Could you check a few things on this model? Use its own coordinates, in mm. Face numbers are marked on the shaded views. A direction names the side the tool comes from. Coordinates: 2 decimals unless noted, no trailing zeros. Order: outer loops, then holes, each group sorted by start corner. A loop starts at its lowest first (then second) coordinate and runs counter-clockwise, first axis right, second up. Notation, with made-up numbers: M 28,-27.75 L 35,-27.75 A8 ccw 35,-15.75 Z; hole C -35.75,-27 d9. An arc over 180 degrees is marked long. One line per question, with ' | ' between items. Start each with the question number.
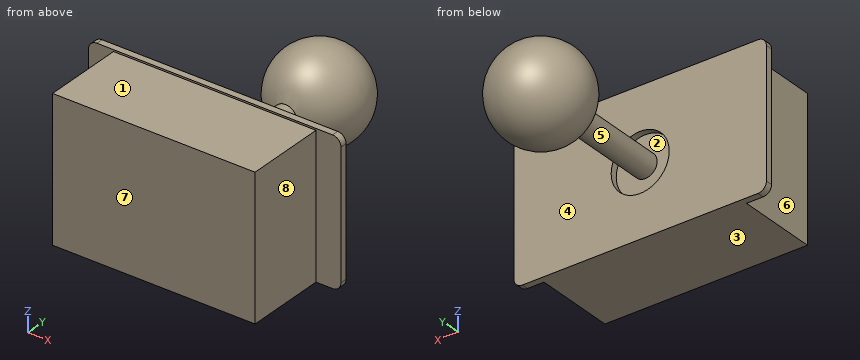
Autodesk Inventor part; units mm, degrees
ref_plane "YZ Plane" through (0, 0, 0) normal (1, 0, 0) x (0, 1, 0)
ref_plane "XZ Plane" through (0, 0, 0) normal (0, 1, 0) x (-1, 0, 0)
ref_plane "XY Plane" through (0, 0, 0) normal (0, 0, 1) x (1, 0, 0)
sketch "Sketch1" plane through (0, 0, 0) normal (0, 1, 0) x (-1, 0, 0)
  line L0 (0, 0) -> (95, 0)
  line L1 (95, 0) -> (95, -54)
  line L2 (95, -54) -> (0, -54)
  line L3 (0, -54) -> (0, 0)
  dimension "d0" = 95
  dimension "d1" = 54
extrude "Extrusion1" add sketch "Sketch1" along normal blind 2.54
fillet "Fillet1" radius 3.175 4 edges at (0, 1.27, 0) (-95, 1.27, 0) (0, 1.27, -54) (-95, 1.27, -54)
sketch "Sketch2" plane through (0, 0, 0) normal (0, -1, 0) x (1, 0, 0)
  arc A0 (-95, -50.825) -> (-91.825, -54) centre (-91.825, -50.825) ccw
  line L0 (-91.825, -54) -> (-3.175, -54)
  arc A1 (-3.175, -54) -> (0, -50.825) centre (-3.175, -50.825) ccw
  line L1 (0, -50.825) -> (0, -3.175)
  arc A2 (0, -3.175) -> (-3.175, 0) centre (-3.175, -3.175) ccw
  line L2 (-3.175, 0) -> (-91.825, 0)
  arc A3 (-91.825, 0) -> (-95, -3.175) centre (-91.825, -3.175) ccw
  line L3 (-95, -3.175) -> (-95, -50.825)
  line L4 (-85.602, -54) -> (-9.402, -54)
  line L5 (-9.402, -54) -> (-9.402, -0.66)
  line L6 (-9.402, -0.66) -> (-85.602, -0.66)
  line L7 (-85.602, -0.66) -> (-85.602, -54)
  point P0 (0, 0)
  dimension "d5" = 76.2
  dimension "d6" = 53.34
  dimension "d7" = 0
  dimension "d8" = 9.398
extrude "Extrusion2" add sketch "Sketch2" along normal blind 30.48 contours L7 L6 L5 L0
sketch "Sketch3" plane through (0, 2.54, 0) normal (0, 1, 0) x (1, 0, 0)
  arc A0 (-91.825, 54) -> (-95, 50.825) centre (-91.825, 50.825) ccw
  arc A1 (-91.825, 54) -> (-95, 50.825) centre (-91.825, 50.825) ccw
  line L0 (-95, 50.825) -> (-95, 3.175)
  arc A2 (-95, 3.175) -> (-91.825, 0) centre (-91.825, 3.175) ccw
  line L1 (-91.825, 0) -> (-3.175, 0)
  arc A3 (-3.175, 0) -> (0, 3.175) centre (-3.175, 3.175) ccw
  line L2 (0, 3.175) -> (0, 50.825)
  arc A4 (0, 50.825) -> (-3.175, 54) centre (-3.175, 50.825) ccw
  line L3 (-3.175, 54) -> (-91.825, 54)
  line L4 (-3.175, 3.175) -> (-91.825, 50.825)
  circle A5 centre (-47.5, 27) radius 10.922
  point P0 (0, 0)
  dimension "d11" = 21.844
extrude "Extrusion3" cut sketch "Sketch3" against normal blind 2.54 contours A5 L4 | L4 A5
sketch "Sketch4" plane through (-47.5, 0, -27) normal (0, 1, 0) x (1, 0, 0)
  circle A0 centre (0, 0) radius 4.4704
  point P0 (47.5, -27)
  dimension "d14" = 8.9408
extrude "Extrusion4" add sketch "Sketch4" along normal blind 43.815
ref_plane "Work Plane1" through (-47.5, 52.315, -27) normal (0, 1, 0) x (1, 0, 0)
sketch "Sketch5" plane through (-47.5, 52.315, -27) normal (0, 1, 0) x (1, 0, 0)
  arc A0 (-17.5, 0) -> (17.5, 0) centre (0, 0) ccw
  line L0 (17.5, 0) -> (-17.5, 0)
  point P0 (47.5, -27)
  dimension "d18" = 35
revolve "Revolution1" add sketch "Sketch5" angle 360 about axis through (-30, 52.315, -27) along (-1, 0, 0)
properties part number "Joy_Stick"
(1) We'd pull the mould along Z, two halves only. Please class the marked faces 1, 2, 3 and 4: +Z half, -Z half, draft (parallel to the pull), parting line (faces both ways), or undercut.
(2) Imagine slicing it at B-B, the plane z = -27. Write out the boundary of the cut face in (x, y) (3 decimals), plus the area to 3 significant figures.
(3) Imagine slicing it at C-C, the plane x = -47.5. Write out the boundary of the cut face in (y, z) (3 decimals).
(4) On a 3-axis mill with a long thin cutter (end or side, diameter ignored), from which of +Z, -Z, +X, -X, +Y, -Y can I reach the whole of each face in a straight line? I mean the marked faces 5, 6, 7 and 8. Say none if no direction works.
(5) If I drill on line 1 along Z through (x, y) = (-47.5, 1.05); line 2 along X through (y, z) = (0.6, -27); line 3 along Z through (x, y) = (-47, 1), over which ranges is the centre line in solid material (lowest first)? Write a range as from..to.
(6) For P1, Ø2, axis at x = -12.5, z = -30.5, coming from the +Y side; P2, Ø1.5, axis at x = -54, y = 38.5, coming from the +Z side; P3, Ø13, axis at x = -47.5, z = -27, coming from the +Y side (3 decimals), each with a flat end and sliding along its axis, tell me the tip position at first contact or that it passes through.
(7) Imagine slicing it at A-A, the plane x = -32.5. Write out the boundary of the cut face in (y, z) (3 decimals).
(8) Imagine slicing it at D-D, the plane x = -60. Write out the boundary of the cut face in (y, z) (3 decimals).
Answers:
1) face 1: +Z half | face 2: undercut | face 3: -Z half | face 4: draft
2) outline: M -95,0 L -85.602,0 L -85.602,-30.48 L -9.402,-30.48 L -9.402,0 L 0,0 L 0,2.54 L -36.578,2.54 L -36.578,0 L -43.03,0 L -43.03,35.396 A17.5 ccw long -51.97,35.396 L -51.97,0 L -58.422,0 L -58.422,2.54 L -95,2.54 Z | area: 3,780 mm²
3) outline: M -30.48,-54 L 2.54,-54 L 2.54,-37.922 L 0,-37.922 L 0,-31.47 L 35.396,-31.47 A17.5 ccw long 35.396,-22.53 L 0,-22.53 L 0,-16.078 L 2.54,-16.078 L 2.54,0 L 0,0 L 0,-0.66 L -30.48,-0.66 Z
4) face 5: none | face 6: +Z, -Z, -X, -Y | face 7: +Z, -Z, +X, -X, -Y | face 8: +Z, -Z, +X, -Y
5) line 1: -54..-37.92, -31.47..-22.53, -16.08..0 | line 2: -95..-58.42, -51.97..-43.03, -36.58..0 | line 3: -54..-37.91, -31.44..-22.56, -16.09..0
6) P1: y = 2.54 | P2: z = -17.23 | P3: y = 69.815
7) outline: M -30.48,-54 L 2.54,-54 L 2.54,0 L 0,0 L 0,-0.66 L -30.48,-0.66 Z; C 52.315,-27 d18.028
8) outline: M -30.48,-54 L 2.54,-54 L 2.54,0 L 0,0 L 0,-0.66 L -30.48,-0.66 Z; C 52.315,-27 d24.495
